Can you work these out from the model? Positions are in its coordinate system, mm. A direction names the side the tool comes from. Round coordinates to 2 decimals unless told otherwise and drop trailing zeros. Write each loop counter-clockwise with the first axis right and the second up, starting at its lowest first coordinate (ties: lowest second). Pieces come first, ordered by that corner, then holes. Notation, with made-up numbers: M 24.25,40.25 L 75.25,40.25 A19 ccw 75.25,55.25 Z; hole C -17.5,-8 d1. An arc over 180 degrees is marked long. Answer as a JSON object with one key per item and string values. Group by question number.
1) On a 3-axis mill with a long thin cutter (end or side, diameter ignored), from which of +Z, -Z, +X, -X, +Y, -Y can I reach the whole of each face in a straight line? I mean faces 1 (the cylindrical face through (12.932, -5.362, 13.699)), 2 (the flat face through (0, 0, 9.974)), 3 (the cylindrical face through (-20.597, -16.288, 10.706)). Say none if no direction works.
2) I'm going to push flat-ended pins straight in: pin 1 Ø18 at (x, y) = (0, 0) entering from -Z; pin 2 Ø1 at (x, z) = (3.5, 16.5) entering from +Y; pin 3 Ø1.5 at (x, y) = (-10.5, -8) entering from +Z. Where does each tip first touch, or does it pass through?
3) Suppose I cut it at C-C, the plane x = -17. Write out the boundary of the cut face in (y, z).
4) Please list where these lines run through material, in increasing order: L1, parallel to Y at x = 17.5, z = 11.2; L2, parallel to Z at x = -10, y = -9; L3, parallel to Z at x = -19, y = -6. Write a range as [from, to].
5) Suppose I cut it at D-D, the plane z = 18.5. Write out the boundary of the cut face in (x, y) (3 decimals).
6) Suppose I cut it at B-B, the plane y = 0. Write out the boundary of the cut face in (x, z) (3 decimals), and give its area (3 significant figures).
7) If we mould it in two halves opening along X, with no side actions, what happens to faces 4 (the cylindrical face through (-17.728, -12.265, 10.706)), 5 (the flat face through (21.875, 0, 11)), 6 (the cylindrical face through (-1.873, 0.082, 19.932))? For each: +X half, -X half, draft (parallel to the pull), parting line (faces both ways), or undercut.
8) Suppose I cut it at A-A, the plane x = 0. Write out the boundary of the cut face in (y, z) (3 decimals).
from build123d import *

# Parameters (mm, degrees)
SKETCH1_R           = 7
BOSS_EXTRUDE1_DEPTH = 10
SKETCH2_R           = 56
BOSS_EXTRUDE2_DEPTH = 20
SKETCH3_R           = 3
SKETCH4_R           = 7.5
BOSS_EXTRUDE3_DEPTH = 25
CHAMFER1_SIZE       = 1
SKETCH5_R           = 45
CUT_EXTRUDE1_DEPTH  = 2
SCALE1_SCALE        = 0.25


with BuildPart() as part:
    # Sketch1 → Boss-Extrude1 (new body)
    with BuildSketch(Plane.XY):
        with BuildLine():
            Line((-70.5, 70), (70.5, 70))
            ThreePointArc((70.5, 70), (82.52081528, 65.02081528), (87.5, 53))
            Line((87.5, 53), (87.5, -53))
            ThreePointArc((87.5, -53), (82.52081528, -65.02081528), (70.5, -70))
            Line((70.5, -70), (-70.5, -70))
            ThreePointArc((-70.5, -70), (-82.52081528, -65.02081528), (-87.5, -53))
            Line((-87.5, -53), (-87.5, 53))
            ThreePointArc((-87.5, 53), (-82.52081528, 65.02081528), (-70.5, 70))
        make_face()
        with Locations((-70, 56)):
            Circle(SKETCH1_R, mode=Mode.SUBTRACT)
        with Locations((-70, -56)):
            Circle(SKETCH1_R, mode=Mode.SUBTRACT)
        with Locations((70, -56)):
            Circle(SKETCH1_R, mode=Mode.SUBTRACT)
        with Locations((70, 56)):
            Circle(SKETCH1_R, mode=Mode.SUBTRACT)
    extrude(amount=BOSS_EXTRUDE1_DEPTH)

    # Sketch2 → Boss-Extrude2 (add)
    with BuildSketch(Plane.XY.offset(10)):
        Circle(SKETCH2_R)
    extrude(amount=BOSS_EXTRUDE2_DEPTH)

    # Sketch3 → Revolve1 (revolve)
    with BuildSketch(Plane(origin=(0, 0, 0), x_dir=(1, 0, 0), z_dir=(0, 1, 0)), mode=Mode.PRIVATE) as revolve1_sk:
        with Locations((-56, -27)):
            Circle(SKETCH3_R)
    revolve(revolve1_sk.sketch.rotate(Axis((0, 0, 0), (0, 0, 1)), 180), axis=Axis((0, 0, 0), (0, 0, 1)))

    # Sketch4 → Boss-Extrude3 (add)
    with BuildSketch(Plane.XY.offset(30)):
        Circle(SKETCH4_R)
    extrude(amount=BOSS_EXTRUDE3_DEPTH)

    # Chamfer1
    chamfer1_edges = [part.edges().sort_by_distance(p)[0] for p in [
        (-7.5, 0, 55),
    ]]
    chamfer(chamfer1_edges, length=CHAMFER1_SIZE)

    # Sketch5 → Cut-Extrude1 (cut)
    with BuildSketch(Plane(origin=(0, 0, 0), x_dir=(-1, 0, 0), z_dir=(0, 0, -1))):
        Circle(SKETCH5_R)
    extrude(amount=-CUT_EXTRUDE1_DEPTH, mode=Mode.SUBTRACT)


with BuildPart() as part_1:
    # Scale1: scaled about (0, 0, 12.631964086)
    add(part.part.scale(SCALE1_SCALE).moved(Location((0, 0, 9.473973065))))


solid = part_1.part
Results:
{
 "1": {"face 1": "none", "face 2": "-Z", "face 3": "+Z, -Z, -X, -Y"},
 "2": {"pin 1": "z = 9.97", "pin 2": "y = 14.43", "pin 3": "z = 16.97"},
 "3": {"outline": "M -17.5,9.47 L -15.68,9.47 L -15.68,11.97 L -17.5,11.97 Z; M -12.32,9.47 L 12.32,9.47 L 12.32,11.97 L -12.32,11.97 Z; M 15.68,9.47 L 17.5,9.47 L 17.5,11.97 L 15.68,11.97 Z"},
 "4": {"L1": "[-17.5, -15.75], [-12.25, 12.25], [15.75, 17.5]", "L2": "[9.47, 16.97]", "L3": "[9.47, 11.97]"},
 "5": {"outline": "C 0,0 d3.75"},
 "6": {"outline": "M -21.875,9.474 L -11.25,9.474 L -11.25,9.974 L 11.25,9.974 L 11.25,9.474 L 21.875,9.474 L 21.875,11.974 L 14,11.974 L 14,15.474 A0.75 ccw 14,16.974 L 1.875,16.974 L 1.875,22.974 L 1.625,23.224 L -1.625,23.224 L -1.875,22.974 L -1.875,16.974 L -14,16.974 A0.75 ccw -14,15.474 L -14,11.974 L -21.875,11.974 Z", "area": "263 mm^2"},
 "7": {"face 4": "undercut", "face 5": "+X half", "face 6": "parting line"},
 "8": {"outline": "M -17.5,9.474 L -11.25,9.474 L -11.25,9.974 L 11.25,9.974 L 11.25,9.474 L 17.5,9.474 L 17.5,11.974 L 14,11.974 L 14,15.474 A0.75 ccw 14,16.974 L 1.875,16.974 L 1.875,22.974 L 1.625,23.224 L -1.625,23.224 L -1.875,22.974 L -1.875,16.974 L -14,16.974 A0.75 ccw -14,15.474 L -14,11.974 L -17.5,11.974 Z"}
}
